from build123d import *

# Parameters (mm, degrees)
F1_DEPTH     = 25
F2_R         = 15.5
F3_DEPTH     = 10
F4_T1_DEPTH  = 34.6410161514
F4_T3_DEPTH  = 34.6410161514
F4_T5_DEPTH  = 34.6410161514
F4_T8_ANGLE  = 120
F4_T10_ANGLE = 120
F4_T12_ANGLE = 120


# Not quite as in the source:
# - a fillet or chamfer that OpenCascade refuses, or shapes differently, is made with other operations: its cross-section is extruded or revolved along the edge and cut away or added


with BuildPart() as f1:
    # F0 (on Top) → F1 (new body)
    with BuildSketch(Plane.XY):
        with BuildLine():
            Line((17.3205080757, 30), (-17.3205080757, 30))
            ThreePointArc((-17.3205080757, 30), (-34.6410161514, 20), (-34.6410161514, 0))
            Line((-34.6410161514, 0), (-17.3205080757, -30))
            ThreePointArc((-17.3205080757, -30), (0, -40), (17.3205080757, -30))
            Line((17.3205080757, -30), (34.6410161514, 0))
            ThreePointArc((34.6410161514, 0), (34.6410161514, 20), (17.3205080757, 30))
        make_face()
    extrude(amount=F1_DEPTH)

    # F2 (on face) → F3 (cut)
    with BuildSketch(Plane.XY.offset(25)):
        with Locations((-17.3205080757, 10)):
            Circle(F2_R)
        with Locations((0, -20)):
            Circle(F2_R)
        with Locations((17.3205080757, 10)):
            Circle(F2_R)
    extrude(amount=-F3_DEPTH, mode=Mode.SUBTRACT)

    # F4: chamfer of 5 on 1 edges, made by hand

    # F4_s2 → F4_t1 (cut)
    with BuildSketch(Plane(origin=(-8.6602540378, -15, 0), x_dir=(0, 0, 1), z_dir=(0.5, 0.8660254038, 0))):
        Polygon((25, 25), (20, 30), (25, 30), align=None)
    extrude(amount=F4_T1_DEPTH, mode=Mode.SUBTRACT)

    # F4_s4 → F4_t3 (cut)
    with BuildSketch(Plane.YZ.offset(-17.3205080757)):
        Polygon((30, 20), (25, 25), (30, 25), align=None)
    extrude(amount=F4_T3_DEPTH, mode=Mode.SUBTRACT)

    # F4_s6 → F4_t5 (cut)
    with BuildSketch(Plane(origin=(-8.6602540378, 15, 0), x_dir=(0, 0, 1), z_dir=(0.5, -0.8660254038, 0))):
        Polygon((25, 25), (20, 30), (25, 30), align=None)
    extrude(amount=F4_T5_DEPTH, mode=Mode.SUBTRACT)

    # F4_s7 → F4_t8 (revolve, cut)
    with BuildSketch(Plane(origin=(8.6602540378, -15, 0), x_dir=(0, 0, 1), z_dir=(-0.5, 0.8660254038, 0))):
        Polygon((25, -25), (20, -30), (25, -30), align=None)
    revolve(axis=Axis((0, -20, 25), (0, 0, 1)), revolution_arc=F4_T8_ANGLE, mode=Mode.SUBTRACT)

    # F4_s9 → F4_t10 (revolve, cut)
    with BuildSketch(Plane(origin=(8.6602540378, 15, 0), x_dir=(0, 0, 1), z_dir=(-0.5, -0.8660254038, 0))):
        Polygon((20, -30), (25, -25), (25, -30), align=None)
    revolve(axis=Axis((17.3205080757, 10, 25), (0, 0, 1)), revolution_arc=F4_T10_ANGLE, mode=Mode.SUBTRACT)

    # F4_s11 → F4_t12 (revolve, cut)
    with BuildSketch(Plane.YZ.offset(-17.3205080757)):
        Polygon((30, 20), (25, 25), (30, 25), align=None)
    revolve(axis=Axis((-17.3205080757, 10, 25), (0, 0, 1)), revolution_arc=F4_T12_ANGLE, mode=Mode.SUBTRACT)


solid = f1.part
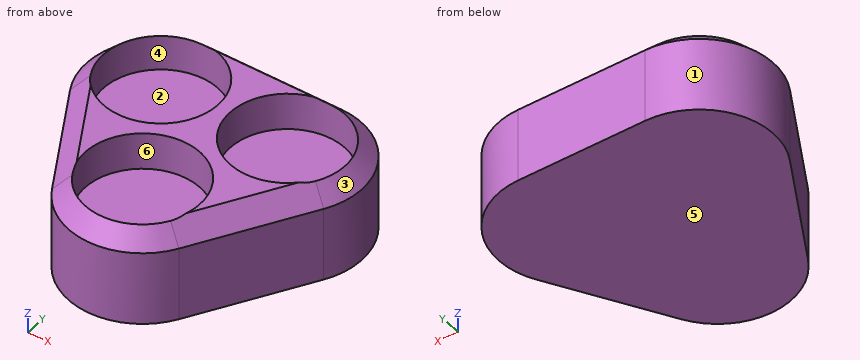
Could you check a few things on this model? Use its own coordinates, in mm. Face numbers are marked on the shaded views. A direction names the side the tool comes from. Give positions to 0.01 mm unless a question says otherwise; leave off trailing zeros. Order: outer loops, then holes, each group sorted by start corner. A loop starts at its lowest first (then second) coordinate and runs counter-clockwise, first axis right, second up. Notation, with made-up numbers: (-11.5, -15.75) -> (3.5, -15.75) arc R14 cw to (3.5, 1.25) -> close; hole circle Ø6 at (50.25, 15). An arc over 180 degrees is marked (long way). Answer in a Markdown table with one row per item. Add a question column.
Item 1: Imagine slicing it at B-B (z = 22.5). List the corners of the cut face in (x, y) for me, and give its area (3 significant figures).
Item 2: Imagine slicing it at D-D (z = 9). List the corners of the cut face in (x, y) for me.
Item 3: Please list where these lines run through material, in increasing order: probe 1 along X at (y, z) = (10, 18.75); probe 2 along Y at (x, z) = (-7, 16.5) (3 decimals); probe 3 along X at (y, z) = (14.5, 19.25).
Item 4: Imagine slicing it at A-A (y = 10). List the corners of the cut face in (x, z) for me.
Item 5: For the marked faces 1 and 2, which set-ups out of +Z, -Z, +X, -X, +Y, -Y let a thin tool reach every point of the face, with its end or its side?
Item 6: Imagine slicing it at C-C (x = 0). List the corners of the cut face in (y, z) for me.
Item 7: I'm going to push flat-ended pins straight in: P1, Ø3, axis at x = -20.5, z = 13.5, coming from the -Y side; P2, Ø10, axis at x = -24, y = 16.5, coming from the +Z side; P3, Ø1.5, axis at y = 3.5, z = 7.5, coming from the -X side. Where does each tip first touch, or does it pass through?
Item 8: We'd pull the mould along Y, two halves only. Please class the marked faces 3, 4, 5 and 6: pulls with the +Y half, pulls with the -Y half, needs draft (parallel to the pull), parting line crosses it, or undercut.
Result:
| question | item | result |
|---|---|---|
| 1 | outline | (-32.48, 1.25) -> (-15.16, -28.75) arc R17.5 ccw to (15.16, -28.75) -> (32.48, 1.25) arc R17.5 ccw to (17.32, 27.5) -> (-17.32, 27.5) arc R17.5 ccw to start; hole circle Ø31 at (-17.32, 10); hole circle Ø31 at (0, -20); hole circle Ø31 at (17.32, 10) |
| 1 | area | 1,040 mm2 |
| 2 | outline | (-34.64, 0) -> (-17.32, -30) arc R20 ccw to (17.32, -30) -> (34.64, 0) arc R20 ccw to (17.32, 30) -> (-17.32, 30) arc R20 ccw to start |
| 3 | probe 1 | -37.32 to -32.82, -1.82 to 1.82, 32.82 to 37.32 |
| 3 | probe 2 | -38.735 to -33.829, -6.171 to -1.564, 21.564 to 30 |
| 3 | probe 3 | -36.81 to -32.15, -2.49 to 2.49, 32.15 to 36.81 |
| 4 | outline | (-37.32, 0) -> (37.32, 0) -> (37.32, 20) -> (32.82, 24.5) -> (32.82, 15) -> (1.82, 15) -> (1.82, 25) -> (-1.82, 25) -> (-1.82, 15) -> (-32.82, 15) -> (-32.82, 24.5) -> (-37.32, 20) -> close |
| 5 | face 1 | +Z, -Z, -X |
| 5 | face 2 | +Z |
| 6 | outline | (-40, 0) -> (30, 0) -> (30, 20) -> (25, 25) -> (-4.5, 25) -> (-4.5, 15) -> (-35.5, 15) -> (-35.5, 24.5) -> (-40, 20) -> close |
| 7 | P1 | y = -27.09 |
| 7 | P2 | z = 15 |
| 7 | P3 | x = -36.48 |
| 8 | face 3 | parting line crosses it |
| 8 | face 4 | undercut |
| 8 | face 5 | needs draft |
| 8 | face 6 | undercut |
